Here's how the part is built. I have some questions about the finished solid (model axes, mm). A direction names the side the tool comes from. Give positions to 0.01 mm unless a question says otherwise; leave off trailing zeros. Loops run counter-clockwise (first coordinate to the right, second up) from the corner with the lowest first, then second, coordinate; pieces in that order, holes last. Notation, with made-up numbers: (-39.5, -31.75) - (2.5, -31.75) arc R9 ccw to (2.5, -22.75) - close; hole circle Ø1 at (66, 14.5). An arc over 180 degrees is marked (long way). Use a Markdown table: item, result.
from build123d import *

# Parameters (mm, degrees)
SKETCH_1_R          = 17.28
SKETCH_1_R_2        = 5.5
SKETCH_1_R_3        = 2.65
SKETCH_1_R_4        = 1.9
EXTRUDE_1_DEPTH     = 3.8
SKETCH_2_R          = 2.5
CUT_EXTRUDE_1_DEPTH = 25.731291919
SKETCH_3_R          = 17.28
SKETCH_3_R_2        = 5.5
SKETCH_3_R_3        = 2.5
SKETCH_3_R_4        = 0.9
EXTRUDE_2_DEPTH     = 2.2


with BuildPart() as part:
    # 草图1 → 凸台-拉伸1 (new body)
    with BuildSketch(Plane(origin=(0, 0, 0), x_dir=(1, 0, 0), z_dir=(0, 1, 0))):
        with Locations(Location((0, 0, 0), (0, 0, 90))):
            Circle(SKETCH_1_R)
        with Locations(Location((0, 0, 0), (0, 0, 90))):
            Circle(SKETCH_1_R_2, mode=Mode.SUBTRACT)
        with Locations(Location((-10, 5.678908346, 0), (0, 0, 90))):
            Circle(SKETCH_1_R_3, mode=Mode.SUBTRACT)
        with Locations(Location((-6.595, -9.561091654, 0), (0, 0, 90))):
            Circle(SKETCH_1_R_4, mode=Mode.SUBTRACT)
        with Locations(Location((6.595, -9.561091654, 0), (0, 0, 90))):
            Circle(SKETCH_1_R_4, mode=Mode.SUBTRACT)
        with Locations(Location((10, 5.678908346, 0), (0, 0, 90))):
            Circle(SKETCH_1_R_3, mode=Mode.SUBTRACT)
    extrude(amount=EXTRUDE_1_DEPTH)

    # 草图2 → 切除-拉伸1 (cut, through all)
    with BuildSketch(Plane(origin=(0, 3.8, 0), x_dir=(1, 0, 0), z_dir=(0, 1, 0))):
        with Locations(Location((-4.85, 9.644699566, 0), (0, 0, 270))):
            Circle(SKETCH_2_R)
    extrude(amount=-CUT_EXTRUDE_1_DEPTH, mode=Mode.SUBTRACT)

    # 草图3 → 凸台-拉伸2 (add)
    with BuildSketch(Plane(origin=(0, 3.8, 0), x_dir=(1, 0, 0), z_dir=(0, 1, 0))):
        with Locations(Location((0, 0, 0), (0, 0, 90))):
            Circle(SKETCH_3_R)
        with Locations(Location((0, 0, 0), (0, 0, 90))):
            Circle(SKETCH_3_R_2, mode=Mode.SUBTRACT)
        with Locations(Location((-4.85, 9.644699566, 0), (0, 0, 270))):
            Circle(SKETCH_3_R_3, mode=Mode.SUBTRACT)
        with Locations(Location((-6.595, -9.561091654, 0), (0, 0, 270))):
            Circle(SKETCH_3_R_4, mode=Mode.SUBTRACT)
        with Locations(Location((6.595, -9.561091654, 0), (0, 0, 90))):
            Circle(SKETCH_3_R_4, mode=Mode.SUBTRACT)
        with BuildLine():
            Line((-12.309220648, 4.378908346), (-7.690779352, 4.378908346))
            ThreePointArc((-7.690779352, 4.378908346), (-7.35, 5.678908346), (-7.690779352, 6.978908346))
            Line((-7.690779352, 6.978908346), (-12.309220648, 6.978908346))
            ThreePointArc((-12.309220648, 6.978908346), (-12.65, 5.678908346), (-12.309220648, 4.378908346))
        make_face(mode=Mode.SUBTRACT)
        with BuildLine():
            Line((12.309220648, 4.378908346), (7.690779352, 4.378908346))
            ThreePointArc((7.690779352, 4.378908346), (7.35, 5.678908346), (7.690779352, 6.978908346))
            Line((7.690779352, 6.978908346), (12.309220648, 6.978908346))
            ThreePointArc((12.309220648, 6.978908346), (12.65, 5.678908346), (12.309220648, 4.378908346))
        make_face(mode=Mode.SUBTRACT)
    extrude(amount=EXTRUDE_2_DEPTH)


solid = part.part
(1) Suppose I cut it at C-C on y = 1.65. Write out the boundary of the cut face in (x, z) (3 decimals).
A:
| item | result |
|---|---|
| outline | circle Ø34.56 at (0, 0); hole circle Ø5.3 at (-10, -5.679); hole circle Ø3.8 at (-6.595, 9.561); hole circle Ø5 at (-4.85, -9.645); hole circle Ø11 at (0, 0); hole circle Ø3.8 at (6.595, 9.561); hole circle Ø5.3 at (10, -5.679) |
(2) Suppose I cut it at A-A on z = 0. Write out the boundary of the cut face in (x, y), plus the area to 3 significant figures.
A:
| item | result |
|---|---|
| outline | (-17.28, 0) - (-5.5, 0) - (-5.5, 6) - (-17.28, 6) - close; (5.5, 0) - (17.28, 0) - (17.28, 6) - (5.5, 6) - close |
| area | 141 mm2 |
(3) Suppose I cut it at D-D on x = 10. Write out the boundary of the cut face in (y, z).
A:
| item | result |
|---|---|
| outline | (0, -14.09) - (6, -14.09) - (6, -6.98) - (3.8, -6.98) - (3.8, -8.33) - (0, -8.33) - close; (0, -3.03) - (3.8, -3.03) - (3.8, -4.38) - (6, -4.38) - (6, 14.09) - (0, 14.09) - close |
(4) Suppose I cut it at B-B on x = 0. Write out the boundary of the cut face in (y, z), plus the area to 3 significant figures.
A:
| item | result |
|---|---|
| outline | (0, -17.28) - (6, -17.28) - (6, -5.5) - (0, -5.5) - close; (0, 5.5) - (6, 5.5) - (6, 17.28) - (0, 17.28) - close |
| area | 141 mm2 |
(5) Will these pins go through, and if not, where does the flat tip stop? pin 1 (3.5 mm diameter, centred on x = -6.6, z = 9.56, fed in from -Y); pin 2 (1.8 mm diameter, centred on x = -9, y = 4.5, fed in from +Z); pin 3 (2.5 mm diameter, centred on x = -9.5, y = 5, fed in from -Z).
A:
| item | result |
|---|---|
| pin 1 | y = 3.8 |
| pin 2 | z = 15.26 |
| pin 3 | z = -15.18 |
(6) If I drill on line 1 (X direction, y = 3.5, z = 9.5); line 2 (X direction, y = 1.35, z = 0); line 3 (Y direction, x = -9, z = -3.5), over which ranges is the centre line in solid material (lowest first)?
A:
| item | result |
|---|---|
| line 1 | -14.43 to -8.49, -4.7 to 4.7, 8.49 to 14.43 |
| line 2 | -17.28 to -5.5, 5.5 to 17.28 |
| line 3 | 3.8 to 6 |
(7) On a 3-axis mill with a long thin cutter (end or side, diameter ignored), from which of +Z, -Z, +X, -X, +Y, -Y can I reach the whole of each face in a straight line? I mean faces 1 (the face through (-10, 5, -6.979)), 2 (the face through (-10, 3.8, -4)), 3 (the face through (-4, 0, 4)). Say none if no direction works.
A:
| item | result |
|---|---|
| face 1 | +Y, -Y |
| face 2 | -Y |
| face 3 | +Z, -Z, +X, -X, -Y |
(8) We'd pull the mould along X, two halves only. Please class faces 4 (the face through (-4, 6, 4)), 5 (the face through (10, 5, -6.979)), 6 (the face through (-5.19, 2.958, -16.482)): pulls with the +X half, pulls with the -X half, needs draft (parallel to the pull), parting line crosses it, or undercut.
A:
| item | result |
|---|---|
| face 4 | needs draft |
| face 5 | undercut |
| face 6 | parting line crosses it |
